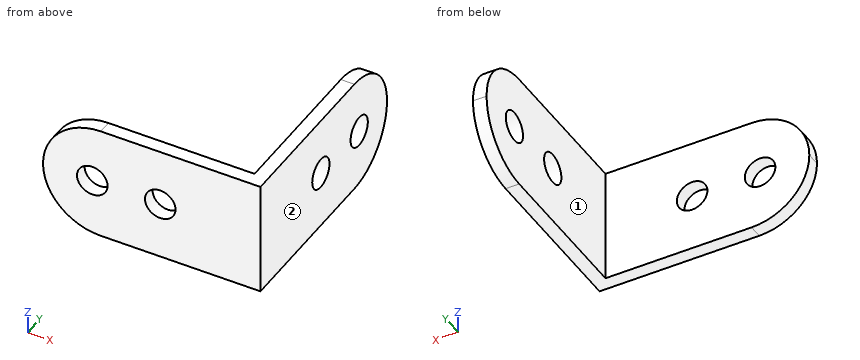
```python
from build123d import *

# Parameters (mm, degrees)
BOSS_EXTRU_1_DEPTH      = 17
ENL_V_MAT_EXTRU_1_DEPTH = 48.728398255
ENL_V_MAT_EXTRU_2_DEPTH = 48.68647607
ESQUISSE4_R             = 2.25
ENL_V_MAT_EXTRU_3_DEPTH = 48.728398255
ESQUISSE5_R             = 2.25
ENL_V_MAT_EXTRU_4_DEPTH = 48.68647607


with BuildPart() as part:
    # Esquisse1 → Boss.-Extru.1 (new body)
    with BuildSketch(Plane.XY):
        Polygon((0, 0), (32, 0), (32, 33), (30, 33), (30, 2), (0, 2), align=None)
    extrude(amount=BOSS_EXTRU_1_DEPTH)

    # Esquisse2 → Enlèv. mat.-Extru.1 (cut, through all)
    with BuildSketch(Plane.ZY.offset(-30)):
        with BuildLine():
            ThreePointArc((8.5, 33), (14.51040764, 30.51040764), (17, 24.5))
            Line((17, 24.5), (17, 33))
            Line((17, 33), (8.5, 33))
        make_face()
        with BuildLine():
            Line((0, 33), (0, 24.5))
            ThreePointArc((0, 24.5), (2.48959236, 30.51040764), (8.5, 33))
            Line((8.5, 33), (0, 33))
        make_face()
    extrude(amount=-ENL_V_MAT_EXTRU_1_DEPTH, mode=Mode.SUBTRACT)

    # Esquisse3 → Enlèv. mat.-Extru.2 (cut, through all)
    with BuildSketch(Plane(origin=(0, 2, 0), x_dir=(1, 0, 0), z_dir=(0, 1, 0))):
        with BuildLine():
            ThreePointArc((8.5, -17), (2.48959236, -14.51040764), (0, -8.5))
            Line((0, -8.5), (0, -17))
            Line((0, -17), (8.5, -17))
        make_face()
        with BuildLine():
            ThreePointArc((0, -8.5), (2.48959236, -2.48959236), (8.5, 0))
            Line((8.5, 0), (0, 0))
            Line((0, 0), (0, -8.5))
        make_face()
    extrude(amount=-ENL_V_MAT_EXTRU_2_DEPTH, mode=Mode.SUBTRACT)

    # Esquisse4 → Enlèv. mat.-Extru.3 (cut, through all)
    with BuildSketch(Plane.ZY.offset(-30)):
        with Locations(Location((8.5, 25.75, 0), (0, 0, 270))):
            Circle(ESQUISSE4_R)
        with Locations(Location((8.5, 15.75, 0), (0, 0, 270))):
            Circle(ESQUISSE4_R)
    extrude(amount=-ENL_V_MAT_EXTRU_3_DEPTH, mode=Mode.SUBTRACT)

    # Esquisse5 → Enlèv. mat.-Extru.4 (cut, through all)
    with BuildSketch(Plane(origin=(0, 2, 0), x_dir=(1, 0, 0), z_dir=(0, 1, 0))):
        with Locations(Location((7.25, -8.5, 0), (0, 0, 180))):
            Circle(ESQUISSE5_R)
        with Locations(Location((17.25, -8.5, 0), (0, 0, 180))):
            Circle(ESQUISSE5_R)
    extrude(amount=-ENL_V_MAT_EXTRU_4_DEPTH, mode=Mode.SUBTRACT)


solid = part.part
```
CAD build for the part. Positions are in the model's coordinates, mm. Face numbers are marked on the shaded views. A direction names the side the tool comes from. Round coordinates to 2 decimals unless told otherwise and drop trailing zeros. Loops run counter-clockwise (first coordinate to the right, second up) from the corner with the lowest first, then second, coordinate; pieces in that order, holes last. Notation, with made-up numbers: M 26,68 L 65,68 A21 ccw 65,101 Z; hole C 46.5,44.5 d8. An arc over 180 degrees is marked long. Return JSON: item names as keys, results as strings. Group by question number.
(1) Tool access for the marked faces 1 and 2: list every direction of +Z, -Z, +X, -X, +Y, -Y with a clear straight run to the whole face (end or side of a thin tool).
(2) Drop flat-ended pins along their axis: P1, Ø8, axis at y = 8, z = 12, coming from the -X side; P2, Ø3.5, axis at y = 25.75, z = 8.5, coming from the +X side; P3, Ø6, axis at x = 15, z = 12, coming from the -Y side; P4, Ø1, axis at x = 13, z = 10, coming from the +Y side. Give the stop position or say it passes through.
(3) Saw through at C-C, the plane y = 3. List the corners of the cut face in (x, z), and give its area (3 significant figures).
(4) Saw through at B-B, the plane x = 17.25. List the corners of the cut face in (y, z), and give its area (3 significant figures).
(5) Saw through at D-D, the plane z = 5.5. List the corners of the cut face in (x, y), and give its area (3 significant figures).
(6) Saw through at A-A, the plane y = 15.75. List the corners of the cut face in (x, z), and give its area (3 significant figures).
(7) Wall check: probe 1 along Z at (x, y) = (17.25, 1.45); probe 2 along Y at (x, z) = (28, 1.5); probe 3 along X at (y, z) = (11.5, 4.5). Give the ranges that are in metal, low to high. Write a range as [from, to].
Answer list:
{
 "1": {"face 1": "+Z, -Z, -X, +Y", "face 2": "+Z, -Z, +X, +Y, -Y"},
 "2": {"P1": "x = 30", "P2": "through", "P3": "y = 0", "P4": "y = 2"},
 "3": {"outline": "M 30,0 L 32,0 L 32,17 L 30,17 Z", "area": "34.0 mm2"},
 "4": {"outline": "M 0,0 L 2,0 L 2,6.25 L 0,6.25 Z; M 0,10.75 L 2,10.75 L 2,17 L 0,17 Z", "area": "25.0 mm2"},
 "5": {"outline": "M 0.55,0 L 32,0 L 32,32.45 L 30,32.45 L 30,2 L 0.55,2 Z", "area": "124 mm2"},
 "6": {"outline": "M 30,0 L 32,0 L 32,6.25 L 30,6.25 Z; M 30,10.75 L 32,10.75 L 32,17 L 30,17 Z", "area": "25.0 mm2"},
 "7": {"probe 1": "[0, 6.25], [10.75, 17]", "probe 2": "[0, 2]", "probe 3": "[30, 32]"}
}
